Print and shaded views of the part. All mm, measured from the part's lowest x, y and z. Coordinates: 2 decimals unless noted, no trailing zeros. Loops run counter-clockwise (first coordinate to the right, second up) from the corner with the lowest first, then second, coordinate; pieces in that order, holes last. Notation, with made-up numbers: M -30,-30.5 L -12,-30.5 A12 ccw -12,-7.5 Z; hole C 61,9.5 d9. An arc over 180 degrees is marked long. Answer as a JSON object with one key per item and string values. Group by question number.
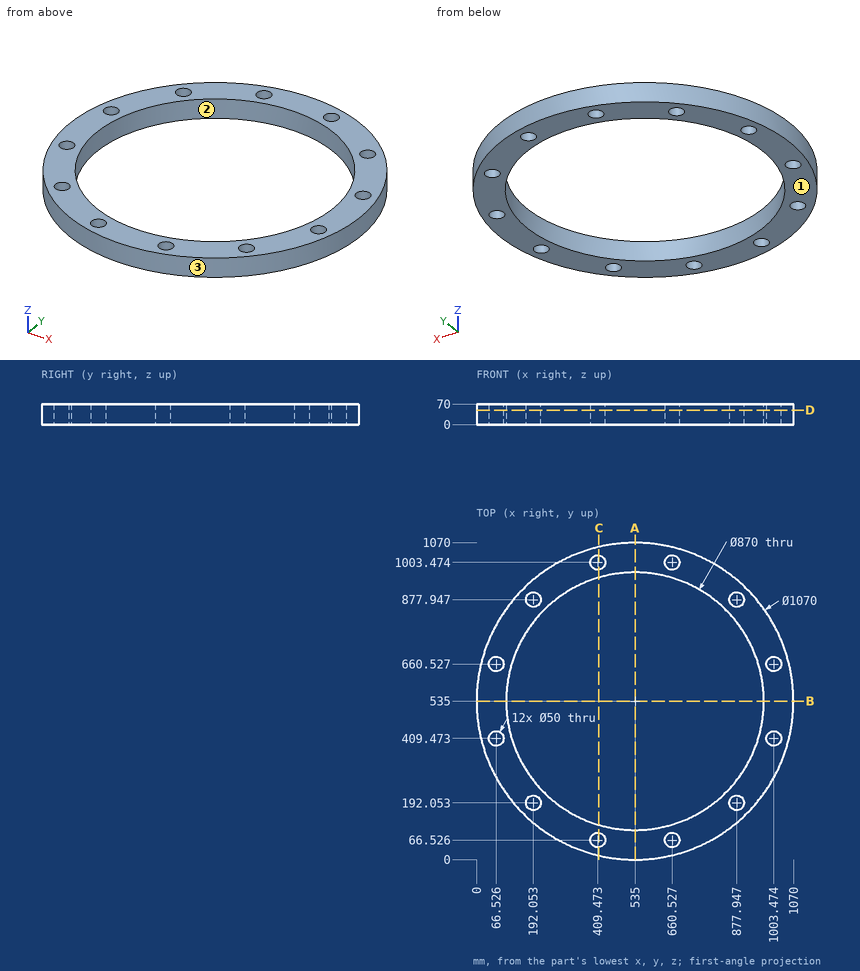
Item 1: Slice it at C-C, the plane x = 413. Write the cut outline in (y, z), then the cut area to 3 significant figures.
Item 2: Slice it at D-D, the plane z = 49. Count the separate pieces of the cut face and the enclosed holes in it, then the cut area to 3 significant figures.
Item 3: Drill centre lines: L1, parallel to X at y = 524, z = 6; L2, parallel to Y at x = 402.5, z = 10.5; L3, parallel to X at y = 856, z = 38.5 (1 decimal). Where is each one in solid material? Low to high. Write a range as from..to.
Item 4: Slice it at A-A, the plane x = 535. Write the cut outline in (y, z), then the cut area to 3 significant figures.
Item 5: Pin check, flat tips, straight feed: pin 1 (1 mm diameter, centred on x = 601.5, z = 45, fed in from +Y); pin 2 (5 mm diameter, centred on x = 172, z = 31, fed in from +Y); pin 3 (2 mm diameter, centred on y = 799.5, z = 17, fed in from -X). Stop position of each tip, or through.
Item 6: Pull direction Y, two halves, no side cores. Call the marked faces 1, 2 and 3: released by +Y, released by -Y, zero draft, split by the parting line, or undercut.
Computed:
{
 "1": {"outline": "M 14.1,0 L 41.78,0 L 41.78,70 L 14.1,70 Z; M 91.28,0 L 117.46,0 L 117.46,70 L 91.28,70 Z; M 952.54,0 L 978.72,0 L 978.72,70 L 952.54,70 Z; M 1028.22,0 L 1055.9,0 L 1055.9,70 L 1028.22,70 Z", "area": "7,540 mm2"},
 "2": {"separate pieces": "1", "enclosed holes": "13", "area": "281,000 mm2"},
 "3": {"L1": "0.11..100.14, 969.86..1069.89", "L2": "16.67..42.52, 90.53..120.67, 949.33..979.47, 1027.48..1053.33", "L3": "107..180.1, 204..241.4, 828.6..866, 889.9..963"},
 "4": {"outline": "M 0,0 L 100,0 L 100,70 L 0,70 Z; M 970,0 L 1070,0 L 1070,70 L 970,70 Z", "area": "14,000 mm2"},
 "5": {"pin 1": "y = 1065.91", "pin 2": "y = 930.3", "pin 3": "x = 69.39"},
 "6": {"face 1": "zero draft", "face 2": "undercut", "face 3": "split by the parting line"}
}
